```python
from build123d import *

# Parameters (mm, degrees)
ESQUISSE1_W             = 25
ESQUISSE1_H             = 12
ESQUISSE1_R             = 2.2
BOSS_EXTRU_1_DEPTH      = 4
ESQUISSE5_W             = 25
ESQUISSE5_H             = 2
BOSS_EXTRU_2_DEPTH      = 17
ESQUISSE6_R             = 0.9
ENL_V_MAT_EXTRU_1_DEPTH = 17
CONG_2_R                = 2


with BuildPart() as part:
    # Esquisse1 → Boss.-Extru.1 (new body)
    with BuildSketch(Plane(origin=(0, 0, 0), x_dir=(1, 0, 0), z_dir=(0, 1, 0))):
        with Locations((0, 1.258064516)):
            Rectangle(ESQUISSE1_W, ESQUISSE1_H)
        with Locations(Location((9, -0.741935484, 0), (0, 0, 270))):
            Circle(ESQUISSE1_R, mode=Mode.SUBTRACT)
        with Locations(Location((-9, -0.741935484, 0), (0, 0, 270))):
            Circle(ESQUISSE1_R, mode=Mode.SUBTRACT)
    extrude(amount=BOSS_EXTRU_1_DEPTH)

    # Esquisse5 → Boss.-Extru.2 (add, along a direction that is not the sketch's normal)
    with BuildSketch(Plane(origin=(0, 4, 0), x_dir=(1, 0, 0), z_dir=(0, 1, 0))):
        with Locations((0, 6.258064516)):
            Rectangle(ESQUISSE5_W, ESQUISSE5_H)
    extrude(amount=BOSS_EXTRU_2_DEPTH, dir=(0, 0.9975640502598248, 0.06975647374411817))

    # Esquisse6 → Enlèv. mat.-Extru.1 (cut)
    with BuildSketch(Plane(origin=(0, 0.385354434, -5.510825157), x_dir=(1, 0, 0), z_dir=(0, -0.06975647374411817, 0.9975640502598248))):
        with Locations(Location((-9.75, 18.940348686, 0), (0, 0, 270))):
            Circle(ESQUISSE6_R)
        with Locations(Location((9.75, 18.940348686, 0), (0, 0, 270))):
            Circle(ESQUISSE6_R)
    extrude(amount=-ENL_V_MAT_EXTRU_1_DEPTH, mode=Mode.SUBTRACT)

    # Congé2
    cong_2_edges = [part.edges().sort_by_distance(p)[0] for p in [
        (0, 4, -5.258064516),
    ]]
    fillet(cong_2_edges, radius=CONG_2_R)


solid = part.part
```
Read the model definition and answer for the solid it produces. Units are mm, in the model's axes. A direction names the side the tool comes from. Round coordinates to 2 decimals unless told otherwise and drop trailing zeros. Write each loop counter-clockwise with the first axis right and the second up, starting at its lowest first coordinate (ties: lowest second). Pieces come first, ordered by that corner, then holes. Notation, with made-up numbers: (-4, -22.75) - (33, -22.75) arc R23 cw to (33, -13.75) - close; hole circle Ø10 at (89.25, 87.25). An arc over 180 degrees is marked (long way). One line per item, written item: value.
Q1. Find section B-B (x = -2). Determine the outline of the cut face in (y, z), and give its area (3 significant figures).
The answers:
outline: (0, -7.26) - (4, -7.26) - (20.96, -6.07) - (20.96, -4.07) - (6.14, -5.11) arc R2 cw to (4, -3.11) - (4, 4.74) - (0, 4.74) - close
area: 82.9 mm2
Q2. For a pull along X with two mould halves and no side action, classify faces 1 (the flat face through (-12.5, 7, -6)), 2 (the cylindrical face through (9.66, 1.97, 2.84)), 3 (the flat face through (-0.175, 12.361, -6.673)) as pulls with the +X half, pulls with the -X half, needs draft (parallel to the pull), parting line crosses it, or undercut.
The answers:
face 1: pulls with the -X half
face 2: undercut
face 3: needs draft
Q3. Straight lines are drawn through the part: line 1 (Y direction, x = -1, z = 4.25); line 2 (Z direction, x = -11, y = 8.25); line 3 (Z direction, x = 7.5, y = 18.25). For each, find the intervals that lie inside material, in ascending order. Write a range as from..to.
The answers:
line 1: y = 0..4
line 2: z = -6.96..-4.96
line 3: z = -6.26..-4.26
Q4. Which of the six approach directions +Z, -Z, +X, -X, +Y, -Y give full straight-line access (tool end or side, diameter ignored) to faces 4 (the cylindrical face through (0.18, 4.65, -4.59)), 5 (the flat face through (0, 4, 1)), 6 (the cylindrical face through (-8.99, 18.87, -5.2))?
The answers:
face 4: +Z, +X, -X
face 5: +Z, +X, -X, +Y
face 6: none
Q5. Find section C-C (x = 7.5). Determine the outline of the cut face in (y, z), and give its area (3 significant figures).
The answers:
outline: (0, -7.26) - (4, -7.26) - (20.96, -6.07) - (20.96, -4.07) - (6.14, -5.11) arc R2 cw to (4, -3.11) - (4, -0.87) - (0, -0.87) - close; (0, 2.35) - (4, 2.35) - (4, 4.74) - (0, 4.74) - close
area: 70.1 mm2
Q6. Find section A-A (z = 0.75). Determine the outline of the cut face in (x, y), and give its area (3 significant figures).
The answers:
outline: (-12.5, 0) - (-11.2, 0) - (-11.2, 4) - (-12.5, 4) - close; (-6.8, 0) - (6.8, 0) - (6.8, 4) - (-6.8, 4) - close; (11.2, 0) - (12.5, 0) - (12.5, 4) - (11.2, 4) - close
area: 64.8 mm2
Q7. Find section D-D (y = 19.5). Count the separate pieces of the cut face and the enclosed holes in it, and give its area (3 significant figures).
The answers:
separate pieces: 3
enclosed holes: 0
area: 42.9 mm2
Q8. Each of these flat-tipped pins is pushed along its axis until it touches: P1, Ø1, axis at x = -4.5, y = 10.5, coming from the +Z side; P2, Ø2.5, axis at x = -1.5, z = -1, coming from the +Y side; P3, Ø2, axis at x = -9.5, y = 5.5, coming from the +Z side. Where does it stop, or does it pass through?
The answers:
P1: stops at z = -4.77
P2: stops at y = 4
P3: stops at z = -4.44
